Read the model definition and answer for the solid it produces. Units are mm, in the model's axes. A direction names the side the tool comes from. Give positions to 0.01 mm unless a question says otherwise; leave off trailing zeros. Order: outer loops, then holes, each group sorted by start corner. A loop starts at its lowest first (then second) coordinate and runs counter-clockwise, first axis right, second up. Notation, with made-up numbers: (8, -26.75) - (59, -26.75) arc R14 cw to (59, -20.75) - close; hole circle Ø1 at (-16, -9.5). An arc over 180 degrees is marked (long way). Write each question's results on one line, items separated by ' | '.
from build123d import *

# Parameters (mm, degrees)
SKETCH1_R           = 25
SKETCH1_R_2         = 1.5
SKETCH1_R_3         = 15
BOSS_EXTRUDE1_DEPTH = 3
SKETCH2_R           = 3.25
CUT_EXTRUDE1_DEPTH  = 2


with BuildPart() as part:
    # Sketch1 → Boss-Extrude1 (new body)
    with BuildSketch(Plane(origin=(0, 0, 0), x_dir=(1, 0, 0), z_dir=(0, 1, 0))):
        with Locations(Location((0, 0, 0), (0, 0, 270))):
            Circle(SKETCH1_R)
        with Locations(Location((0, 20.5, 0), (0, 0, 270))):
            Circle(SKETCH1_R_2, mode=Mode.SUBTRACT)
        with Locations(Location((17.753520778, -10.25, 0), (0, 0, 270))):
            Circle(SKETCH1_R_2, mode=Mode.SUBTRACT)
        with Locations(Location((-17.753520778, -10.25, 0), (0, 0, 270))):
            Circle(SKETCH1_R_2, mode=Mode.SUBTRACT)
        with Locations(Location((0, 0, 0), (0, 0, 270))):
            Circle(SKETCH1_R_3, mode=Mode.SUBTRACT)
    extrude(amount=BOSS_EXTRUDE1_DEPTH)

    # Sketch2 → Cut-Extrude1 (cut)
    with BuildSketch(Plane(origin=(0, 3, 0), x_dir=(1, 0, 0), z_dir=(0, 1, 0))):
        with Locations(Location((0, 20.5, 0), (0, 0, 270))):
            Circle(SKETCH2_R)
        with Locations(Location((17.753520778, -10.25, 0), (0, 0, 270))):
            Circle(SKETCH2_R)
        with Locations(Location((-17.753520778, -10.25, 0), (0, 0, 270))):
            Circle(SKETCH2_R)
    extrude(amount=-CUT_EXTRUDE1_DEPTH, mode=Mode.SUBTRACT)


solid = part.part
(1) Section A-A (x = 0) is taken. Give the vertices of the cut face in (y, z).
Conclusion:
outline: (0, -25) - (3, -25) - (3, -23.75) - (1, -23.75) - (1, -22) - (0, -22) - close; (0, -19) - (1, -19) - (1, -17.25) - (3, -17.25) - (3, -15) - (0, -15) - close; (0, 15) - (3, 15) - (3, 25) - (0, 25) - close
(2) Section B-B (z = 0) is taken. Give the vertices of the cut face in (x, y), plus the area to 3 significant figures.
Conclusion:
outline: (-25, 0) - (-15, 0) - (-15, 3) - (-25, 3) - close; (15, 0) - (25, 0) - (25, 3) - (15, 3) - close | area: 60.0 mm^2
(3) For faces 4 (the face through (17, 1, 12)), 5 (the face through (0.66, 1.479, -14.985)), determine the directions among +Z, -Z, +X, -X, +Y, -Y from which every point of the face is accessible in a straight line to the end or side of a thin tool.
Conclusion:
face 4: +Y | face 5: +Y, -Y
(4) Section D-D (z = 10.25) is taken. Give the vertices of the cut face in (x, y), plus the area to 3 significant figures.
Conclusion:
outline: (-22.8, 0) - (-19.25, 0) - (-19.25, 1) - (-21, 1) - (-21, 3) - (-22.8, 3) - close; (-16.25, 0) - (-10.95, 0) - (-10.95, 3) - (-14.5, 3) - (-14.5, 1) - (-16.25, 1) - close; (10.95, 0) - (16.25, 0) - (16.25, 1) - (14.5, 1) - (14.5, 3) - (10.95, 3) - close; (19.25, 0) - (22.8, 0) - (22.8, 3) - (21, 3) - (21, 1) - (19.25, 1) - close | area: 39.1 mm^2
(5) The mould has two halves that part along X. Classify faces 1 (the face through (-11, 0, 11)), 2 (the face through (7.509, 1.479, 23.846)), 3 (the face through (-1, 1, -19)): pulls with the +X half, pulls with the -X half, needs draft (parallel to the pull), parting line crosses it, or undercut.
Conclusion:
face 1: needs draft | face 2: parting line crosses it | face 3: undercut
(6) Consider probe 1 along X at (y, z) = (1.55, 10.25); probe 2 along X at (y, z) = (0.85, 0); probe 3 along X at (y, z) = (0.45, 10.25). Determine where each line is inside the solid, lowest interval first. Write a range as [from, to].
Conclusion:
probe 1: [-22.8, -21], [-14.5, -10.95], [10.95, 14.5], [21, 22.8] | probe 2: [-25, -15], [15, 25] | probe 3: [-22.8, -19.25], [-16.25, -10.95], [10.95, 16.25], [19.25, 22.8]
(7) Each of these flat-tipped pins is pushed along its axis until it touches: pin 1 (3 mm diameter, centred on x = -16.5, z = 10.5, fed in from +Y); pin 2 (1.5 mm diameter, centred on y = 1.5, z = -2.5, fed in from -X). Where does it stop, or does it pass through?
Conclusion:
pin 1: y = 1 | pin 2: x = -24.94
(8) Section C-C (x = 11) is taken. Give the vertices of the cut face in (y, z), plus the area to 3 significant figures.
Conclusion:
outline: (0, -22.45) - (3, -22.45) - (3, -10.2) - (0, -10.2) - close; (0, 10.2) - (3, 10.2) - (3, 22.45) - (0, 22.45) - close | area: 73.5 mm^2
